Design review of the part built by this model. Coordinates are the model's own, in mm. A direction names the side the tool comes from. Coordinates: 2 decimals unless noted, no trailing zeros. Write each loop counter-clockwise with the first axis right and the second up, starting at its lowest first coordinate (ties: lowest second). Pieces come first, ordered by that corner, then holes. Notation, with made-up numbers: (72, 22.5) - (114, 22.5) arc R13 ccw to (114, 28.5) - close; hole circle Ø2 at (26, 65.5). An arc over 180 degrees is marked (long way). Answer as a JSON object with one key per item and string values.
```python
from build123d import *

# Parameters (mm, degrees)
F0_W     = 36.5
F0_H     = 60.22
F1_DEPTH = 7
F2_W     = 4
F2_H     = 7
F3_DEPTH = 2
F4_R     = 2


with BuildPart() as f1:
    # F0 (on Top) → F1 (new body)
    with BuildSketch(Plane.XY):
        Rectangle(F0_W, F0_H)
    extrude(amount=F1_DEPTH)

    # F2 (on face) → F3 (join)
    with BuildSketch(Plane(origin=(0, 30.11, 0), x_dir=(-1, 0, 0), z_dir=(0, 1, 0))):
        with Locations((0, 3.5)):
            Rectangle(F2_W, F2_H)
    extrude(amount=F3_DEPTH)

    # F4
    f4_edges = [f1.edges().sort_by_distance(p)[0] for p in [
        (18.25, 0, 7),
        (18.25, 0, 0),
        (-18.25, 0, 7),
        (-18.25, 0, 0),
    ]]
    fillet(f4_edges, radius=F4_R)


solid = f1.part
```
(1) To check wall thickness, follow line 1 (Y direction, x = 5, z = 5.75); line 2 (X direction, y = 16, z = 1.75); line 3 (X direction, y = -22, z = 6.5). State the ranges of each line that lie inside material, in increasing order. Write a range as from..to.
Solved:
{"line 1": "y = -30.11..30.11", "line 2": "x = -18.23..18.23", "line 3": "x = -17.57..17.57"}
(2) Tool access review of faces 1 (the face through (-10, 30.11, 3)), 2 (the face through (10, 30.11, 3)), 3 (the face through (0, -30.11, 3)): name each direction out of +Z, -Z, +X, -X, +Y, -Y from which nothing blocks a thin tool from reaching the whole face with its end or side.
Solved:
{"face 1": "+Z, -Z, -X, +Y", "face 2": "+Z, -Z, +X, +Y", "face 3": "+Z, -Z, +X, -X, -Y"}
(3) Take a section at A-A, the plane z = 3.5. Write out the cut boundary in (x, y).
Solved:
{"outline": "(-18.25, -30.11) - (18.25, -30.11) - (18.25, 30.11) - (2, 30.11) - (2, 32.11) - (-2, 32.11) - (-2, 30.11) - (-18.25, 30.11) - close"}
(4) Take a section at B-B, the plane x = 3.5. Write out the cut boundary in (y, z).
Solved:
{"outline": "(-30.11, 0) - (30.11, 0) - (30.11, 7) - (-30.11, 7) - close"}
(5) For pin 1 (0.6 mm diameter, centred on y = 30.5, z = 3.5, fed in from -X); pin 2 (3.5 mm diameter, centred on x = -8.5, z = 4, fed in from +Y); pin 3 (1.6 mm diameter, centred on y = 31, z = 2.5, fed in from +X), all flat-tipped, find the tip position at first contact; note any pin that passes through.
Solved:
{"pin 1": "stops at x = -2", "pin 2": "stops at y = 30.11", "pin 3": "stops at x = 2"}
